Input: dimensioned drawing with shaded views. Units: mm. Origin: part minimum x, y, z. A direction names the side the tool comes from. Round coordinates to 2 decimals unless told otherwise and drop trailing zeros. Loops run counter-clockwise (first coordinate to the right, second up) from the corner with the lowest first, then second, coordinate; pieces in that order, holes last.
Item 1: Section query C-C on y = 3.5. Return loops of the section in (x, z).
Item 2: Access query for the marked faces 1, 2 and 3. Directions: +Z, -Z, +X, -X, +Y, -Y. A direction counts if a zero-diameter tool reaches every point of the face in a straight line with its end or side. Return the directions, or none.
Item 3: Section query D-D on z = 3.4. Return loops of the section in (x, y), then the cut area to 3 significant figures.
Item 4: Section query A-A on x = 2. Return loops of the section in (y, z), then the cut area to 3 significant figures.
Item 5: Section query B-B on z = 2. Return loops of the section in (x, y).
Item 6: First-contact query: P1, Ø0.9, axis at x = 3, y = 7, coming from the +Z side; P2, Ø2, axis at x = 2.5, y = 1.5, coming from the -Z side; P3, Ø1.5, axis at y = 3, z = 3, coming from the -X side. Flat tips, straight axial feed; report the tip coordinate or a pass-through.
Item 7: Pull-direction query (X, two-part tool) for the marked faces 4, 5, 6 and 7; classes: released by +X, released by -X, zero draft, split by the parting line, or undercut.
Item 8: Ray query, L1, parallel to Y at x = 2.6, z = 0.55; L2, parallel to X at y = 7, z = 2.7 (1 decimal); L3, parallel to Y at x = 2.05, z = 1.7. Return the intervals inside material, ascending.
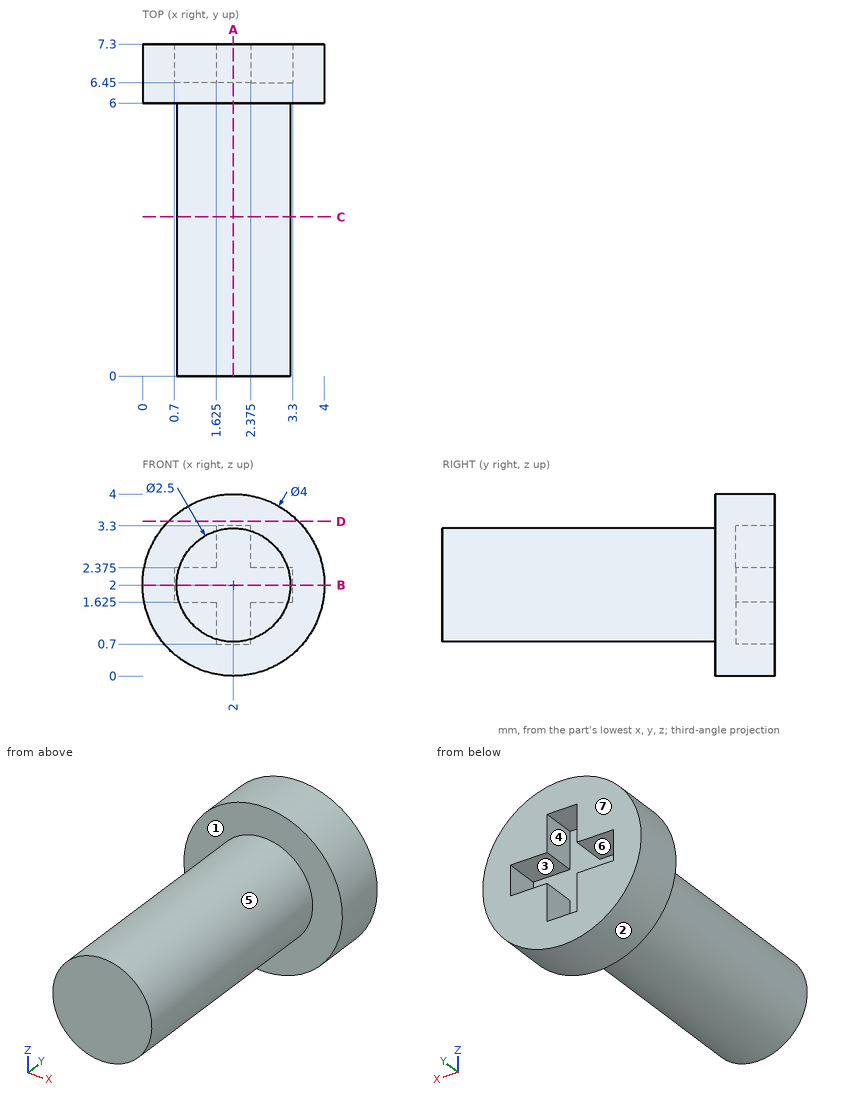
Data:
1. outline: circle Ø2.5 at (2, 2)
2. face 1: -Y
2. face 2: +Y, -Y
2. face 3: +Y
3. outline: (0.57, 6) - (3.43, 6) - (3.43, 7.3) - (0.57, 7.3) - close
3. area: 3.71 mm2
4. outline: (0, 0.75) - (6, 0.75) - (6, 0) - (7.3, 0) - (7.3, 0.7) - (6.45, 0.7) - (6.45, 3.3) - (7.3, 3.3) - (7.3, 4) - (6, 4) - (6, 3.25) - (0, 3.25) - close
4. area: 18.0 mm2
5. outline: (0, 6) - (0.75, 6) - (0.75, 0) - (3.25, 0) - (3.25, 6) - (4, 6) - (4, 7.3) - (3.3, 7.3) - (3.3, 6.45) - (0.7, 6.45) - (0.7, 7.3) - (0, 7.3) - close
6. P1: stops at z = 3.92
6. P2: stops at z = 0.75
6. P3: stops at x = 0.78
7. face 4: undercut
7. face 5: split by the parting line
7. face 6: undercut
7. face 7: zero draft
8. L1: y = 6 to 7.3
8. L2: x = 0.1 to 1.6, 2.4 to 3.9
8. L3: y = 0 to 6.45
